Study the drawing (mm; zero at the part's minimum x, y, z) and answer. A direction names the side the tool comes from. Give positions to 0.01 mm unless a question says otherwise; leave off trailing zeros. Loops run counter-clockwise (first coordinate to the right, second up) from the corner with the lowest first, then second, coordinate; pieces in that order, holes last. Notation, with made-up numbers: M 2,89.25 L 30,89.25 A11 cw 30,106.25 Z; hole C 64,63 d2. An arc over 180 degrees is marked long. Use one line per item in the form item = value. Start each with the question number.
1. The part is cut by section B-B (y = 25.5). Write down the section's boundary in (x, z) (1 decimal), and give its area (3 significant figures).
2. The part is cut by section C-C (x = 19.5). Write down the section's boundary in (y, z) (1 decimal).
3. Each of these flat-tipped pins is pushed along its axis until it touches: pin 1 Ø5 at (x, y) = (18, 22) entering from +Z; pin 2 Ø8 at (x, z) = (17, 31.5) entering from +Y; pin 3 Ø5 at (x, z) = (17.5, 40) entering from -Y; pin 4 Ø8 at (x, z) = (13, 12) entering from -Y. Where does it stop, or does it pass through?
4. For the marked faces 1, 2 and 3, determine the directions among +Z, -Z, +X, -X, +Y, -Y from which every point of the face is accessible in a straight line to the end or side of a thin tool.
5. Straight lines are drawn through the part: line 1 (Y direction, x = 16.5, z = 24) (1 decimal); line 2 (X direction, y = 36.5, z = 4); line 3 (Z direction, x = 19, y = 13) (1 decimal). For each, find the intervals that lie inside material, in ascending order. Write a range as from..to.
6. The part is cut by section D-D (y = 36.5). Write down the section's boundary in (x, z) (1 decimal), and give its area (3 significant figures).
7. The part is cut by section A-A (z = 12.5). Write down the section's boundary in (x, y) (1 decimal).
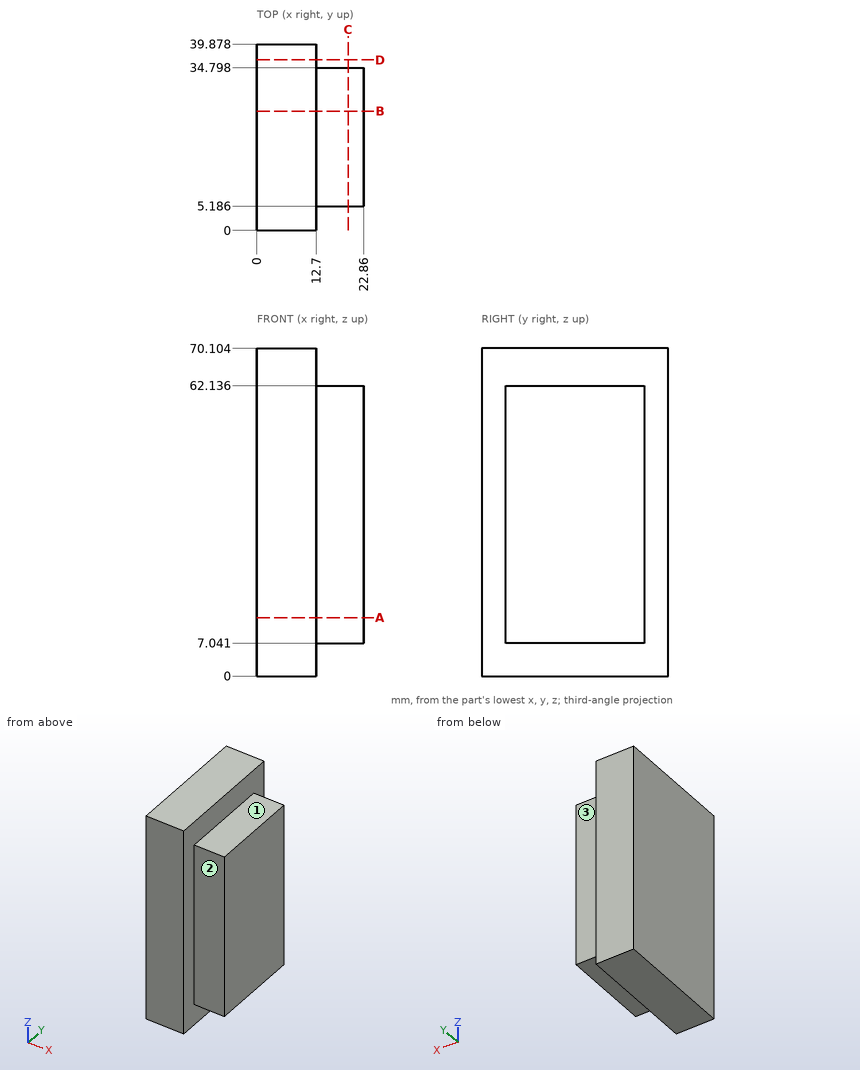
Derived:
q1.outline = M 0,0 L 12.7,0 L 12.7,7 L 22.9,7 L 22.9,62.1 L 12.7,62.1 L 12.7,70.1 L 0,70.1 Z
q1.area = 1,450 mm2
q2.outline = M 5.2,7 L 34.8,7 L 34.8,62.1 L 5.2,62.1 Z
q3.pin_1 = 62.14
q3.pin_2 = 34.8
q3.pin_3 = 5.19
q3.pin_4 = 0
q4.face_1 = +Z, +X, +Y, -Y
q4.face_2 = +Z, -Z, +X, -Y
q4.face_3 = +Z, -Z, +X, +Y
q5.line_1 = 5.2..34.8
q5.line_2 = 0..12.7
q5.line_3 = 7..62.1
q6.outline = M 0,0 L 12.7,0 L 12.7,70.1 L 0,70.1 Z
q6.area = 890 mm2
q7.outline = M 0,0 L 12.7,0 L 12.7,5.2 L 22.9,5.2 L 22.9,34.8 L 12.7,34.8 L 12.7,39.9 L 0,39.9 Z
